from build123d import *

# Parameters (mm, degrees)
SALIENTE_EXTRUIR1_DEPTH      = 3
SALIENTE_EXTRUIR3_DEPTH      = 5
CROQUIS5_W                   = 50
CROQUIS5_H                   = 3
SALIENTE_EXTRUIR4_DEPTH      = 5
SALIENTE_EXTRUIR6_DEPTH      = 5
SALIENTE_EXTRUIR7_DEPTH      = 5
SALIENTE_EXTRUIR7_DEPTH_BACK = 3
CORTAR_EXTRUIR2_DEPTH        = 5
CROQUIS11_R                  = 2
CORTAR_EXTRUIR3_DEPTH        = 5


with BuildPart() as part:
    # Croquis2 → Saliente-Extruir1 (new body)
    with BuildSketch(Plane(origin=(0, 0, 0), x_dir=(1, 0, 0), z_dir=(0, 1, 0))):
        with BuildLine():
            Line((-66.516806956, -7.313551242), (-72, -34.872839919))
            ThreePointArc((-72, -34.872839919), (0, -106.872839919), (72, -34.872839919))
            Line((72, -34.872839919), (66.516806956, -7.313551242))
            ThreePointArc((66.516806956, -7.313551242), (0, 37.127160081), (-66.516806956, -7.313551242))
        make_face()
        with BuildLine():
            Line((-43.798295131, 106.872839919), (-66.516806956, -7.313551242))
            ThreePointArc((-66.516806956, -7.313551242), (0, 37.127160081), (66.516806956, -7.313551242))
            Line((66.516806956, -7.313551242), (43.798295131, 106.872839919))
            Line((43.798295131, 106.872839919), (30, 106.872839919))
            Line((30, 106.872839919), (30, 102.472839919))
            Line((30, 102.472839919), (-30, 102.472839919))
            Line((-30, 102.472839919), (-30, 106.872839919))
            Line((-30, 106.872839919), (-43.798295131, 106.872839919))
        make_face()
    extrude(amount=SALIENTE_EXTRUIR1_DEPTH)

    # Croquis3 → Saliente-Extruir3 (add)
    with BuildSketch(Plane(origin=(0, 3, 0), x_dir=(1, 0, 0), z_dir=(0, 1, 0))):
        with BuildLine():
            Line((0, -100.872839919), (0, -103.372839919))
            ThreePointArc((0, -103.372839919), (13.091100059, -102.110278145), (25.699621359, -98.369134787))
            Line((25.699621359, -98.369134787), (24.761678974, -96.051751763))
            ThreePointArc((24.761678974, -96.051751763), (12.613322685, -99.656357042), (0, -100.872839919))
        make_face()
        with BuildLine():
            ThreePointArc((-25.699621359, -98.369134787), (-13.091100059, -102.110278145), (0, -103.372839919))
            Line((0, -103.372839919), (0, -100.872839919))
            ThreePointArc((0, -100.872839919), (-12.613322685, -99.656357042), (-24.761678974, -96.051751763))
            Line((-24.761678974, -96.051751763), (-25.699621359, -98.369134787))
        make_face()
    extrude(amount=SALIENTE_EXTRUIR3_DEPTH)

    # Croquis5 → Saliente-Extruir4 (add)
    with BuildSketch(Plane(origin=(0, 3, 0), x_dir=(1, 0, 0), z_dir=(0, 1, 0))):
        with Locations((0, 97.772839919)):
            Rectangle(CROQUIS5_W, CROQUIS5_H)
    extrude(amount=SALIENTE_EXTRUIR4_DEPTH)

    # Croquis6 → Saliente-Extruir6 (add)
    with BuildSketch(Plane(origin=(0, 3, 0), x_dir=(1, 0, 0), z_dir=(0, 1, 0))):
        Polygon((-46.298308612, 63.855049889), (-49.044482423, 64.401428328), (-59.164112379, 13.069022297), (-56.507839729, 12.540530583), align=None)
        Polygon((56.507539535, 12.540530583), (46.298008419, 63.855049889), (49.240337502, 64.440455359), (59.449868619, 13.125936053), align=None)
    extrude(amount=SALIENTE_EXTRUIR6_DEPTH)

    # Croquis8 → Saliente-Extruir7 (add, two sides: drawn at the far end of the back side and taken through both)
    with BuildSketch(Plane(origin=(0, 3, 0), x_dir=(1, 0, 0), z_dir=(0, 1, 0)).offset(-SALIENTE_EXTRUIR7_DEPTH_BACK)):
        Polygon((-65.278264707, 14.285493372), (-62.335935624, 13.700087901), (-52.126404507, 65.014607207), (-55.06873359, 65.600012678), align=None)
        Polygon((52.126393076, 65.014664659), (62.335924193, 13.700145353), (65.277964514, 14.285493372), (55.068433397, 65.600012678), align=None)
    extrude(amount=SALIENTE_EXTRUIR7_DEPTH + SALIENTE_EXTRUIR7_DEPTH_BACK)

    # Croquis9 → Cortar-Extruir2 (cut)
    with BuildSketch(Plane(origin=(0, 8, 0), x_dir=(1, 0, 0), z_dir=(0, 1, 0))):
        Polygon((62.335924193, 13.700145353), (62.532079465, 13.739172384), (52.322548348, 65.05369169), (52.126393076, 65.014664659), align=None)
        Polygon((-62.532090896, 13.739114932), (-62.335935624, 13.700087901), (-52.126404507, 65.014607207), (-52.322559779, 65.053634238), align=None)
    extrude(amount=-CORTAR_EXTRUIR2_DEPTH, mode=Mode.SUBTRACT)

    # Croquis11 → Cortar-Extruir3 (cut)
    with BuildSketch(Plane(origin=(0, 3, 0), x_dir=(1, 0, 0), z_dir=(0, 1, 0))):
        with Locations(Location((-0.000150097, 44.590728717, 0), (0, 0, 270))):
            Circle(CROQUIS11_R)
        with Locations(Location((-0.000150097, -45.409271283, 0), (0, 0, 270))):
            Circle(CROQUIS11_R)
    extrude(amount=-CORTAR_EXTRUIR3_DEPTH, mode=Mode.SUBTRACT)


solid = part.part
Read the model definition and answer for the solid it produces. Units are mm, in the model's axes. A direction names the side the tool comes from. Give positions to 0.01 mm unless a question says otherwise; leave off trailing zeros. Write each loop counter-clockwise with the first axis right and the second up, starting at its lowest first coordinate (ties: lowest second). Pieces come first, ordered by that corner, then holes. Notation, with made-up numbers: (18.25, 42.5) - (61.25, 42.5) arc R27 ccw to (61.25, 66.5) - close; hole circle Ø5 at (-5.75, 74.25). An arc over 180 degrees is marked (long way). Answer in a Markdown table with one row per item. Add a question column.
Item 1: A tool of negligible diameter and unlimited length cuts with its end or side. For faces 1 (the face through (0, 5, -96.273)), 2 (the face through (51.474, 5.465, -37.839)), 3 (the face through (-54.033, 5.465, -39.095)), 4 (the face through (58, 8, -40)), from which of +Z, -Z, +X, -X, +Y, -Y can it reach the whole face along a straight path? Write none if from no direction.
Item 2: Section B-B, the plane z = -34 is taken. Write down the section's boundary in (x, y).
Item 3: Section C-C, the plane x = 14.5 is taken. Write down the section's boundary in (y, z).
Item 4: Flat-ended cylindrical pins translate along their axes: P1, Ø3.5, axis at y = 6, z = -97.5, coming from the -X side; P2, Ø1.5, axis at x = -3.5, y = 5.5, coming from the +Z side; P3, Ø2.5, axis at x = -11, y = 4.5, coming from the -Z side; P4, Ø3.5, axis at x = 0, z = -44.59, coming from the -Y side. Find the tip coordinate at first contact, or state that the pin passes through.
Item 5: Find the intervals of material crossed by L1, parallel to X at y = 7.25, z = -27; L2, parallel to X at y = 4.25, z = -31.5; L3, parallel to Y at x = -3, z = -28, in increasing order.
Item 6: Section D-D, the plane x = -6 is taken. Write down the section's boundary in (y, z), and give its area (3 significant figures).
Item 7: Section A-A, the plane y = 5 is taken. Write down the section's boundary in (x, z).
Item 8: Determine the mould class of faces 5 (the face through (0.601, 1.521, 47.317)), 6 (the face through (60.245, 3.944, -39.584)), 7 (the face through (0, 8, 102)), 8 (the face through (-1.583, 1.479, 106.855)) for opening direction X: pulls with the +X half, pulls with the -X half, needs draft (parallel to the pull), parting line crosses it, or undercut.
Recorded:
| question | item | result |
|---|---|---|
| 1 | face 1 | +X, -X, +Y |
| 1 | face 2 | +Z, +Y |
| 1 | face 3 | +Y |
| 1 | face 4 | +Z, -Z, +X, -X, +Y |
| 2 | outline | (-61.36, 0) - (61.36, 0) - (61.36, 8) - (58.5, 8) - (58.5, 3) - (55.3, 3) - (55.3, 8) - (52.24, 8) - (52.24, 3) - (-52.24, 3) - (-52.24, 8) - (-55.04, 8) - (-55.04, 3) - (-58.5, 3) - (-58.5, 8) - (-61.36, 8) - close |
| 3 | outline | (0, -102.47) - (3, -102.47) - (3, -99.27) - (8, -99.27) - (8, -96.27) - (3, -96.27) - (3, 99.26) - (8, 99.26) - (8, 101.82) - (3, 101.82) - (3, 105.4) - (0, 105.4) - close |
| 4 | P1 | stops at x = -25 |
| 4 | P2 | stops at z = 103.32 |
| 4 | P3 | stops at z = -99.27 |
| 4 | P4 | passes through |
| 5 | L1 | x = -62.75 to -59.89, -56.42 to -53.63, 53.63 to 56.69, 59.89 to 62.75 |
| 5 | L2 | x = -61.85 to -59, -55.53 to -52.74, 52.74 to 55.79, 59 to 61.85 |
| 5 | L3 | y = 0 to 3 |
| 6 | outline | (0, -102.47) - (3, -102.47) - (3, -99.27) - (8, -99.27) - (8, -96.27) - (3, -96.27) - (3, 100.6) - (8, 100.6) - (8, 103.11) - (3, 103.11) - (3, 106.62) - (0, 106.62) - close |
| 6 | area | 655 mm2 |
| 7 | outline | (-65.28, -14.29) - (-55.07, -65.6) - (-52.32, -65.05) - (-62.53, -13.74) - close; (-59.16, -13.07) - (-49.04, -64.4) - (-46.3, -63.86) - (-56.51, -12.54) - close; (-25.7, 98.37) - (-24.76, 96.05) arc R66 cw to (24.76, 96.05) - (25.7, 98.37) arc R68.5 ccw to start; (-25, -99.27) - (25, -99.27) - (25, -96.27) - (-25, -96.27) - close; (46.3, -63.86) - (49.24, -64.44) - (59.45, -13.13) - (56.51, -12.54) - close; (52.32, -65.05) - (55.07, -65.6) - (65.28, -14.29) - (62.53, -13.74) - close |
| 8 | face 5 | undercut |
| 8 | face 6 | pulls with the +X half |
| 8 | face 7 | needs draft |
| 8 | face 8 | parting line crosses it |
